from build123d import *

# Parameters (mm, degrees)
SKETCH1_R           = 4.25
SKETCH1_R_2         = 1.75
SKETCH1_R_3         = 0.8
BOSS_EXTRUDE1_DEPTH = 5


with BuildPart() as part:
    # Sketch1 → Boss-Extrude1 (new body)
    with BuildSketch(Plane.XY):
        with BuildLine():
            Line((-18.197591032, 74.9627461), (34.771929891, 68.799966437))
            ThreePointArc((34.771929891, 68.799966437), (42.723806159, 60.240313183), (35.522543907, 51.040214163))
            Line((35.522543907, 51.040214163), (-16.738063779, 40.429894456))
            ThreePointArc((-16.738063779, 40.429894456), (-37.7043906, 56.841024116), (-18.197591032, 74.9627461))
        make_face()
        with Locations((-20.22, 57.58)):
            Circle(SKETCH1_R, mode=Mode.SUBTRACT)
        with Locations((33.73183385, 59.860268443)):
            Circle(SKETCH1_R_2, mode=Mode.SUBTRACT)
        with Locations((-20.22, 66.33)):
            Circle(SKETCH1_R_3, mode=Mode.SUBTRACT)
    extrude(amount=-BOSS_EXTRUDE1_DEPTH)


solid = part.part
The listing builds one solid part. Answer for the finished solid, in the listing's coordinates (mm). Coordinates: 2 decimals unless noted, no trailing zeros. Order: outer loops, then holes, each group sorted by start corner. A loop starts at its lowest first (then second) coordinate and runs counter-clockwise, first axis right, second up. Notation, with made-up numbers: (60, -13) -> (78, -13) arc R23 cw to (78, 14) -> close; hole circle Ø2 at (43, -18). An arc over 180 degrees is marked (long way). Answer in a Markdown table with one row per item. Add a question column.
Item 1: Find section C-C (y = 66.33). Write down the section's boundary in (x, z).
Item 2: Find section D-D (x = 8.5). Write down the section's boundary in (y, z), then the cut area to 3 significant figures.
Item 3: Each of these flat-tipped pins is pushed along its axis until it touches: P1, Ø1, axis at y = 54.5, z = -4, coming from the -X side; P2, Ø1.5, axis at x = -13.5, y = 64, coming from the +Z side; P3, Ø3, axis at x = 17, z = -1, coming from the +Y side; P4, Ø1, axis at x = -27.5, z = -2, coming from the +Y side. Where does it stop, or does it pass through?
Item 4: Find the intervals of material crossed by L1, parallel to Y at x = -20.22, z = -2.35; L2, parallel to X at y = 66.33, z = -3.9; L3, parallel to X at y = 66, z = -3.9, in increasing order. Write a range as from..to.
Item 5: Find section A-A (x = -23.5). Write down the section's boundary in (y, z), then the cut area to 3 significant figures.
Item 6: Find section B-B (z = -2.35). Write down the section's boundary in (x, y).
Item 7: Determine the mould class of faces 1 (the face through (-20.324, 67.123, -2.465)), 2 (the face through (7.916, 71.924, -2.465)), 3 (the face through (34.54, 58.31, -2.46)), 4 (the face through (3, 58, -5)) for opening direction X: +X half, -X half, draft (parallel to the pull), parting line (faces both ways), or undercut.
Result set:
| question | item | result |
|---|---|---|
| 1 | outline | (-35.38, -5) -> (-21.02, -5) -> (-21.02, 0) -> (-35.38, 0) -> close; (-19.42, -5) -> (39.99, -5) -> (39.99, 0) -> (-19.42, 0) -> close |
| 2 | outline | (45.55, -5) -> (71.86, -5) -> (71.86, 0) -> (45.55, 0) -> close |
| 2 | area | 132 mm² |
| 3 | P1 | stops at x = -37.53 |
| 3 | P2 | stops at z = 0 |
| 3 | P3 | stops at y = 71.04 |
| 3 | P4 | stops at y = 73.71 |
| 4 | L1 | y = 40.08..53.33, 61.83..65.53, 67.13..75.08 |
| 4 | L2 | x = -35.38..-21.02, -19.42..39.99 |
| 4 | L3 | x = -35.56..-20.95, -19.49..40.31 |
| 5 | outline | (40.39, -5) -> (54.88, -5) -> (54.88, 0) -> (40.39, 0) -> close; (60.28, -5) -> (74.77, -5) -> (74.77, 0) -> (60.28, 0) -> close |
| 5 | area | 145 mm² |
| 6 | outline | (-18.2, 74.96) arc R17.5 ccw (long way) to (-16.74, 40.43) -> (35.52, 51.04) arc R9 ccw to (34.77, 68.8) -> close; hole circle Ø8.5 at (-20.22, 57.58); hole circle Ø1.6 at (-20.22, 66.33); hole circle Ø3.5 at (33.73, 59.86) |
| 7 | face 1 | undercut |
| 7 | face 2 | +X half |
| 7 | face 3 | undercut |
| 7 | face 4 | draft |
